Check sheet for the modelled part. Datum: model origin and axes. Units: mm. Face numbers are marked on the shaded views. Give positions to 0.01 mm unless a question says otherwise; leave off trailing zeros. Order: outer loops, then holes, each group sorted by start corner. A loop starts at its lowest first (then second) coordinate and runs counter-clockwise, first axis right, second up.
```python
from build123d import *

# Parameters (mm, degrees)
ESBO_O1_W                = 7.6
ESBO_O1_H                = 10.6
ESBO_O1_R                = 1.5
RESSALTO_EXTRUS_O1_DEPTH = 2.6
ESBO_O2_W                = 0.386988846
ESBO_O2_H                = 1.141626943
CORTE_EXTRUS_O1_DEPTH    = 2.4
PADR_OCIRCULAR1_COUNT    = 3
CORTE_EXTRUS_O2_DEPTH    = 0.05
ESBO_O4_W                = 0.8
ESBO_O4_H                = 0.302387696
RESSALTO_EXTRUS_O2_DEPTH = 2.5


with BuildPart() as part:
    # Esboço1 → Ressalto-extrusão1 (new body)
    with BuildSketch(Plane.XY):
        Rectangle(ESBO_O1_W, ESBO_O1_H)
        with Locations((0, 1.5)):
            Circle(ESBO_O1_R, mode=Mode.SUBTRACT)
    extrude(amount=RESSALTO_EXTRUS_O1_DEPTH)

    # Esboço2 → Corte-extrusão1 (cut)
    with BuildSketch(Plane.XY.offset(2.6)):
        with Locations((0, 2.620892828)):
            Rectangle(ESBO_O2_W, ESBO_O2_H)
    corte_extrus_o1 = extrude(amount=-CORTE_EXTRUS_O1_DEPTH, mode=Mode.SUBTRACT)

    # PadrãoCircular1: Corte-extrusão1 ×3 about axis
    padr_ocircular1_axis = Axis((0, 1.5, 0), (0, 0, 1))
    for i in range(1, PADR_OCIRCULAR1_COUNT):
        add(corte_extrus_o1.rotate(padr_ocircular1_axis, i * 360 / PADR_OCIRCULAR1_COUNT), mode=Mode.SUBTRACT)

    # Esboço3 → Corte-extrusão2 (cut)
    with BuildSketch(Plane(origin=(0, 0, 0), x_dir=(-1, 0, 0), z_dir=(0, 0, -1))):
        with BuildLine():
            Line((-1.7, -3.5), (1.7, -3.5))
            ThreePointArc((1.7, -3.5), (2.407106781, -3.207106781), (2.7, -2.5))
            Line((2.7, -2.5), (2.7, 3))
            ThreePointArc((2.7, 3), (2.407106781, 3.707106781), (1.7, 4))
            Line((1.7, 4), (-1.7, 4))
            ThreePointArc((-1.7, 4), (-2.407106781, 3.707106781), (-2.7, 3))
            Line((-2.7, 3), (-2.7, -2.5))
            ThreePointArc((-2.7, -2.5), (-2.407106781, -3.207106781), (-1.7, -3.5))
        make_face()
    extrude(amount=-CORTE_EXTRUS_O2_DEPTH, mode=Mode.SUBTRACT)

    # Esboço4 → Ressalto-extrusão2 (add)
    with BuildSketch(Plane.XZ.offset(5.3)):
        with Locations((-2.54, 1.3)):
            Rectangle(ESBO_O4_W, ESBO_O4_H)
        with Locations((0, 1.3)):
            Rectangle(ESBO_O4_W, ESBO_O4_H)
        with Locations((2.54, 1.3)):
            Rectangle(ESBO_O4_W, ESBO_O4_H)
    extrude(amount=RESSALTO_EXTRUS_O2_DEPTH)


solid = part.part
```
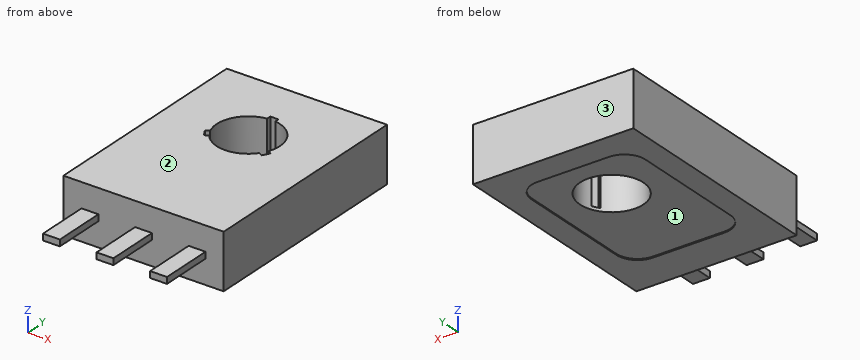
Q1. Go/stop test with flat-tipped pins: P1, Ø2.5, axis at x = -0.5, y = 1.5, coming from the -Z side; P2, Ø1, axis at x = 0.5, y = -6.5, coming from the +Z side; P3, Ø0.9, axis at x = -2.5, y = -7, coming from the -Z side. Record where each tip stops, or that it passes through.
Q2. Sectioned sample at C-C, the plane z = 2.4. Record the cut outline in (x, y), plus the area to 3 significant figures.
Q3. Material ranges on line 1 (Y direction, x = 0, z = 1.5); line 2 (X direction, y = 1.5, z = 0.95); line 3 (Y direction, x = 3.25, z = 0.9), recorded low to high.
Q4. Sectioned sample at B-B, the plane y = 1.5. Record the cut outline in (x, z), plus the area to 3 significant figures.
Q5. Sectioned sample at D-D, the plane y = -6.75. Record the cut outline in (x, z).
Q6. Sectioned sample at A-A, the plane x = 0. Record the cut outline in (y, z).
Q7. Draft check along Y on the marked faces 1, 2 and 3. Enter one of: pulls with the +Y half, pulls with the -Y half, needs draft (parallel to the pull), parting line crosses it, or undercut.
Filled in:
1. P1: stops at z = 0.05
1. P2: stops at z = 1.45
1. P3: stops at z = 1.15
2. outline: (-3.8, -5.3) - (3.8, -5.3) - (3.8, 5.3) - (-3.8, 5.3) - close; hole (-1.56, 0.82) - (-1.37, 0.49) - (-1.19, 0.59) arc R1.5 ccw to (1.19, 0.59) - (1.37, 0.49) - (1.56, 0.82) - (1.38, 0.92) arc R1.5 ccw to (0.19, 2.99) - (0.19, 3.19) - (-0.19, 3.19) - (-0.19, 2.99) arc R1.5 ccw to (-1.38, 0.92) - close
2. area: 73.3 mm2
3. line 1: y = -5.3 to 0, 3.19 to 5.3
3. line 2: x = -3.8 to -1.5, 1.5 to 3.8
3. line 3: y = -5.3 to 5.3
4. outline: (-3.8, 0) - (-2.7, 0) - (-2.7, 0.05) - (-1.5, 0.05) - (-1.5, 2.6) - (-3.8, 2.6) - close; (1.5, 0.05) - (2.7, 0.05) - (2.7, 0) - (3.8, 0) - (3.8, 2.6) - (1.5, 2.6) - close
4. area: 11.8 mm2
5. outline: (-2.94, 1.15) - (-2.14, 1.15) - (-2.14, 1.45) - (-2.94, 1.45) - close; (-0.4, 1.15) - (0.4, 1.15) - (0.4, 1.45) - (-0.4, 1.45) - close; (2.14, 1.15) - (2.94, 1.15) - (2.94, 1.45) - (2.14, 1.45) - close
6. outline: (-7.8, 1.15) - (-5.3, 1.15) - (-5.3, 0) - (-3.5, 0) - (-3.5, 0.05) - (0, 0.05) - (0, 2.6) - (-5.3, 2.6) - (-5.3, 1.45) - (-7.8, 1.45) - close; (3, 0.05) - (4, 0.05) - (4, 0) - (5.3, 0) - (5.3, 2.6) - (3.19, 2.6) - (3.19, 0.2) - (3, 0.2) - close
7. face 1: undercut
7. face 2: needs draft
7. face 3: pulls with the +Y half
